```python
from build123d import *

# Parameters (mm, degrees)
F1_W     = 18
F1_H     = 18
F2_DEPTH = 7.5
F3_DEPTH = 7
F4_R     = 1
F5_DEPTH = 7
F6_R     = 1


with BuildPart() as f2:
    # F1 (on offset) → F2 (new body)
    with BuildSketch(Plane.XY.offset(7.5)):
        with Locations((9, -9)):
            Rectangle(F1_W, F1_H)
        with Locations((-9, 9)):
            Rectangle(F1_W, F1_H)
        with Locations((9, 9)):
            Rectangle(F1_W, F1_H)
        with Locations((-9, -9)):
            Rectangle(F1_W, F1_H)
    extrude(amount=-F2_DEPTH)

    # F1 (on offset) → F3 (cut)
    with BuildSketch(Plane.XY.offset(7.5)):
        with Locations((9, 9)):
            Rectangle(F1_W, F1_H)
    extrude(amount=-F3_DEPTH, mode=Mode.SUBTRACT)

    # F4
    f4_edges = [f2.edges().sort_by_distance(p)[0] for p in [
        (0, 0, 4),
    ]]
    fillet(f4_edges, radius=F4_R)

    # F1 (on offset) → F5 (cut)
    with BuildSketch(Plane.XY.offset(7.5)):
        with Locations((-9, -9)):
            Rectangle(F1_W, F1_H)
    extrude(amount=-F5_DEPTH, mode=Mode.SUBTRACT)

    # F6
    f6_edges = [f2.edges().sort_by_distance(p)[0] for p in [
        (0, 0, 4),
    ]]
    fillet(f6_edges, radius=F6_R)


solid = f2.part
```
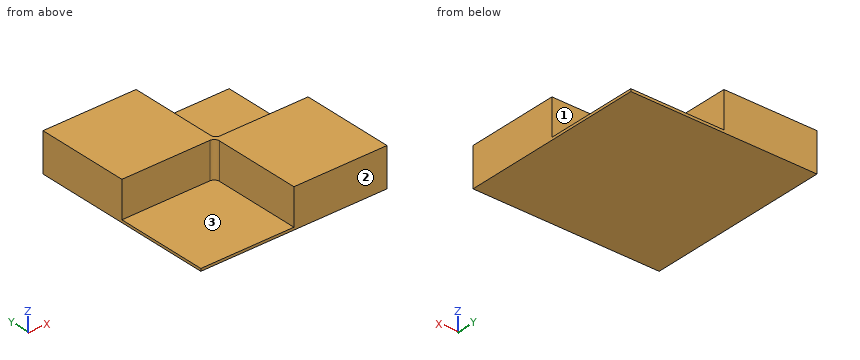
Input: part model. Units: mm. Frame: model coordinates. Face numbers are marked on the shaded views. A direction names the side the tool comes from. Coordinates: 2 decimals unless noted, no trailing zeros. Loops run counter-clockwise (first coordinate to the right, second up) from the corner with the lowest first, then second, coordinate; pieces in that order, holes last. Notation, with made-up numbers: (62.25, 18) -> (120.25, 18) arc R20 ccw to (120.25, 56) -> close; hole circle Ø10 at (65.25, -24.75). An arc over 180 degrees is marked (long way). Use a Markdown table: item, result.
1) Cut plane C-C (y = -13). Return the cut outline in (x, z).
Results found:
| item | result |
|---|---|
| outline | (-18, 0) -> (18, 0) -> (18, 7.5) -> (0, 7.5) -> (0, 0.5) -> (-18, 0.5) -> close |
2) Cut plane B-B (x = 14). Return the cut outline in (y, z), then the cut area to 3 significant figures.
Results found:
| item | result |
|---|---|
| outline | (-18, 0) -> (18, 0) -> (18, 0.5) -> (0, 0.5) -> (0, 7.5) -> (-18, 7.5) -> close |
| area | 144 mm2 |
3) Contact query for flat-ended pins moving along their axis: pin 1 (4 mm diameter, centred on x = 7, z = 3.5, fed in from +Y); pin 2 (9 mm diameter, centred on x = -9.5, y = -9, fed in from +Z); pin 3 (3.5 mm diameter, centred on y = 5.5, z = 3, fed in from +X). Output: stop coordinate, or through.
Results found:
| item | result |
|---|---|
| pin 1 | stops at y = 0 |
| pin 2 | stops at z = 0.5 |
| pin 3 | stops at x = 0 |
4) Access query for the marked faces 1, 2 and 3. Directions: +Z, -Z, +X, -X, +Y, -Y. A direction counts if a zero-diameter tool reaches every point of the face in a straight line with its end or side. Return the directions, or none.
Results found:
| item | result |
|---|---|
| face 1 | +Z, +X, +Y |
| face 2 | +Z, -Z, +X, -X, -Y |
| face 3 | +Z, -X, -Y |
5) Cut plane A-A (z = 5). Return the cut outline in (x, y).
Results found:
| item | result |
|---|---|
| outline | (-18, 0) -> (-1, 0) arc R1 cw to (0, -1) -> (0, -18) -> (18, -18) -> (18, 0) -> (1, 0) arc R1 cw to (0, 1) -> (0, 18) -> (-18, 18) -> close |
6) Material intervals for line 1 along X through (y, z) = (15, 6.75); line 2 along Z through (x, y) = (1, 3); line 3 along Y through (x, z) = (-11, 3), sorted ascending. Write a range as from..to.
Results found:
| item | result |
|---|---|
| line 1 | x = -18..0 |
| line 2 | z = 0..0.5 |
| line 3 | y = 0..18 |
